from build123d import *

# Parameters (mm, degrees)
CHAMFER1_SIZE       = 2.2225
EXTRUDE1_DEPTH      = 71.853025694
EXTRUDE1_DEPTH_BACK = 71.853025694
EXTRUDE3_DEPTH      = 71.853025757
EXTRUDE3_DEPTH_BACK = 71.853025757
SKETCH4_R           = 3.175
EXTRUDE4_DEPTH      = 6.35
EXTRUDE6_DEPTH      = 71.853025757
EXTRUDE6_DEPTH_BACK = 71.853025757
SKETCH6_R           = 5.55625


with BuildPart() as part:
    # Sketch1 → Revolve1 (revolve)
    with BuildSketch(Plane(origin=(0, 0, 0), x_dir=(1, 0, 0), z_dir=(0, 1, 0)), mode=Mode.PRIVATE) as revolve1_sk:
        Polygon((-63.5, 22.225), (-23.01875, 22.225), (11.1125, 22.225), (11.1125, 0), (-63.5, 0), align=None)
    revolve(revolve1_sk.sketch.rotate(Axis((-63.5, 0, 0), (1, 0, 0)), 180), axis=Axis((-63.5, 0, 0), (1, 0, 0)))

    # Chamfer1
    chamfer1_edges = [part.edges().sort_by_distance(p)[0] for p in [
        (11.1125, 0, -22.225),
        (-63.5, 0, -22.225),
    ]]
    chamfer(chamfer1_edges, length=CHAMFER1_SIZE)

    # Sketch2 → Extrude1 (cut, two sides: drawn at the far end of the back side and taken through both)
    with BuildSketch(Plane(origin=(0, 0, 0), x_dir=(1, 0, 0), z_dir=(0, 1, 0)).offset(-EXTRUDE1_DEPTH_BACK)):
        with BuildLine():
            Line((-23.7998, 22.225), (22.225, 22.225))
            Line((22.225, 22.225), (22.225, -22.225))
            Line((22.225, -22.225), (-23.7998, -22.225))
            ThreePointArc((-23.7998, -22.225), (-20.545024106, -14.367275894), (-12.6873, -11.1125))
            Line((-12.6873, -11.1125), (0, -11.1125))
            ThreePointArc((0, -11.1125), (11.1125, 0), (0, 11.1125))
            Line((0, 11.1125), (-12.6873, 11.1125))
            ThreePointArc((-12.6873, 11.1125), (-20.545024106, 14.367275894), (-23.7998, 22.225))
        make_face()
    extrude(amount=EXTRUDE1_DEPTH + EXTRUDE1_DEPTH_BACK, mode=Mode.SUBTRACT)

    # Sketch3 → Extrude3 (cut, two sides: drawn at the far end of the back side and taken through both)
    with BuildSketch(Plane.XY.offset(-EXTRUDE3_DEPTH_BACK)):
        with BuildLine():
            Line((-18.24355, 14.80185), (22.225, 14.80185))
            Line((22.225, 14.80185), (22.225, -14.80185))
            Line((22.225, -14.80185), (-18.24355, -14.80185))
            ThreePointArc((-18.24355, -14.80185), (-23.7998, 0), (-18.24355, 14.80185))
        make_face()
    extrude(amount=EXTRUDE3_DEPTH + EXTRUDE3_DEPTH_BACK, mode=Mode.SUBTRACT)

    # Sketch4 → Extrude4 (cut)
    with BuildSketch(Plane.ZY.offset(63.5)):
        Circle(SKETCH4_R)
    extrude(amount=-EXTRUDE4_DEPTH, mode=Mode.SUBTRACT)

    # Extrude5 cone 1 section (through the dimple's axis) → Extrude5 (revolve, cut)
    with BuildSketch(Plane(origin=(-57.15, 0, 0), x_dir=(0, 0, 1), z_dir=(0, 1, 0))):
        Polygon((0, 0), (3.175, 0), (0, 3.175), align=None)
    revolve(axis=Axis((-57.15, 0, 0), (1, 0, 0)), mode=Mode.SUBTRACT)

    # Sketch6 → Extrude6 (cut, two sides: drawn at the far end of the back side and taken through both)
    with BuildSketch(Plane(origin=(0, 0, 0), x_dir=(1, 0, 0), z_dir=(0, 1, 0)).offset(-EXTRUDE6_DEPTH_BACK)):
        with Locations(Location((0, 0, 0), (0, 0, 270))):
            Circle(SKETCH6_R)
    extrude(amount=EXTRUDE6_DEPTH + EXTRUDE6_DEPTH_BACK, mode=Mode.SUBTRACT)


solid = part.part
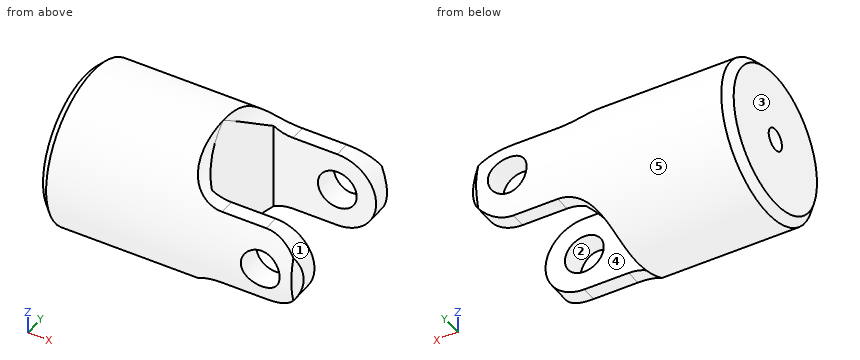
Geometry: final body of the model. Coordinates: model frame, mm. Face numbers are marked on the shaded views. A direction names the side the tool comes from. Round coordinates to 2 decimals unless told otherwise and drop trailing zeros. Loops run counter-clockwise (first coordinate to the right, second up) from the corner with the lowest first, then second, coordinate; pieces in that order, holes last. Notation, with made-up numbers: (-5.5, 44.25) - (-1.5, 44.25) arc R25 cw to (-1.5, 61.25) - close; hole circle Ø9 at (-23.5, 58). An arc over 180 degrees is marked (long way). Write each question's results on one line, items separated by ' | '. Start each with the question number.
1) Line query: probe 1 along Y at (x, z) = (-61.25, 0) (3 decimals); probe 2 along X at (y, z) = (19.75, 0); probe 3 along Y at (x, z) = (-61.75, 0) (1 decimal). Output: solid intervals per line, ascending. Write a range as [from, to].
2) First-contact query: P1, Ø4, axis at y = -12, z = 9.5, coming from the +X side; P2, Ø3.5, axis at x = -6.5, y = -17, coming from the -Z side; P3, Ø10, axis at x = -18.5, y = -11.5, coming from the +Z side; P4, Ø6.5, axis at x = 0, z = 0, coming from the +Y side. Flat tips, straight axial feed; report the tip coordinate or a pass-through.
3) Cut plane B-B on x = -15. Return loops of the section in (y, z) (3 decimals), then the cut area to 3 significant figures.
4) Mould query, pull axis X, two halves, no side actions, for the marked faces 1, 2 and 3. Classes: released by +X, released by -X, zero draft, split by the parting line, or undercut.
5) Cut plane A-A on x = -3.5. Count the separate pieces of the cut face and the enclosed holes in it, then the cut area to 3 significant figures.
6) Access query for the marked faces 4 and 5. Directions: +Z, -Z, +X, -X, +Y, -Y. A direction counts if a zero-diameter tool reaches every point of the face in a straight line with its end or side. Return the directions, or none.
7) Cut plane C-C on x = -30.5. Return loops of the section in (y, z) (3 decimals), then the cut area to 3 significant figures.
Verdict:
1) probe 1: y = [-22.225, -3.175], [3.175, 22.225] | probe 2: x = [-63.5, -5.56], [5.56, 11.11] | probe 3: y = [-21.8, -3.2], [3.2, 21.8]
2) P1: stops at x = -18.91 | P2: stops at z = -11.11 | P3: stops at z = 19.44 | P4: passes through
3) outline: (-19.105, -11.356) - (-14.802, -11.356) - (-14.802, 11.356) - (-19.105, 11.356) arc R22.225 ccw to start; (14.802, -11.356) - (19.105, -11.356) arc R22.225 ccw to (19.105, 11.356) - (14.802, 11.356) - close | area: 291 mm2
4) face 1: released by +X | face 2: undercut | face 3: released by -X
5) separate pieces: 4 | enclosed holes: 0 | area: 161 mm2
6) face 4: +Z, -Z, +X | face 5: +X, -X
7) outline: circle Ø44.45 at (0, 0) | area: 1,550 mm2
